from build123d import *

# Parameters (mm, degrees)
SKETCH1_R           = 1.65
BOSS_EXTRUDE1_DEPTH = 3
BOSS_EXTRUDE2_DEPTH = 16
SKETCH3_R           = 1.65
CUT_EXTRUDE1_DEPTH  = 16
SKETCH5_W           = 10
SKETCH5_H           = 3
BOSS_EXTRUDE3_DEPTH = 14
SKETCH6_R           = 1.65
CUT_EXTRUDE2_DEPTH  = 14


with BuildPart() as part:
    # Sketch1 → Boss-Extrude1 (new body)
    with BuildSketch(Plane(origin=(0, 0, 0), x_dir=(1, 0, 0), z_dir=(0, 1, 0))):
        with BuildLine():
            Line((-10, 70.842692107), (-10, 10))
            Line((-10, 10), (-70.842692107, 10))
            ThreePointArc((-70.842692107, 10), (-71.369207057, 5.012315742), (-71.545, 0))
            ThreePointArc((-71.545, 0), (50.58995466, -50.58995466), (0, 71.545))
            ThreePointArc((0, 71.545), (-5.012315742, 71.369207057), (-10, 70.842692107))
        make_face()
        with Locations((12.13, 16)):
            Circle(SKETCH1_R, mode=Mode.SUBTRACT)
        with Locations((12.13, 54)):
            Circle(SKETCH1_R, mode=Mode.SUBTRACT)
        with Locations((23.25, -21)):
            Circle(SKETCH1_R, mode=Mode.SUBTRACT)
        with Locations((-31.75, -21)):
            Circle(SKETCH1_R, mode=Mode.SUBTRACT)
    extrude(amount=BOSS_EXTRUDE1_DEPTH)

    # Sketch2 → Boss-Extrude2 (add)
    with BuildSketch(Plane.XZ):
        Polygon((-23.600230141, -61.909816502), (53.19593923, -39.496687094), (54.036431583, -42.376543445), (-22.759737789, -64.789672853), align=None)
    extrude(amount=BOSS_EXTRUDE2_DEPTH)

    # Sketch3 → Cut-Extrude1 (cut)
    with BuildSketch(Plane(origin=(14.797854544, 0, -50.703251798), x_dir=(0.959952117, 0, 0.280164118), z_dir=(-0.280164118, 0, 0.959952117))):
        with Locations((-31, -8)):
            Circle(SKETCH3_R)
        with Locations((31, -8)):
            Circle(SKETCH3_R)
    extrude(amount=-CUT_EXTRUDE1_DEPTH, mode=Mode.SUBTRACT)

    # Sketch5 → Boss-Extrude3 (add)
    with BuildSketch(Plane(origin=(0, 0, 0), x_dir=(-1, 0, 0), z_dir=(0, -1, 0))):
        with Locations((0, -63.5)):
            Rectangle(SKETCH5_W, SKETCH5_H)
    extrude(amount=BOSS_EXTRUDE3_DEPTH)

    # Sketch6 → Cut-Extrude2 (cut)
    with BuildSketch(Plane(origin=(0, 0, 62), x_dir=(-1, 0, 0), z_dir=(0, 0, -1))):
        with Locations((0, -7.998816604)):
            Circle(SKETCH6_R)
    extrude(amount=-CUT_EXTRUDE2_DEPTH, mode=Mode.SUBTRACT)


solid = part.part
Model file for the job. Use its own axes, mm. A direction names the side the tool comes from. Give positions to 0.01 mm unless a question says otherwise; leave off trailing zeros. Write each loop counter-clockwise with the first axis right and the second up, starting at its lowest first coordinate (ties: lowest second). Pieces come first, ordered by that corner, then holes. Notation, with made-up numbers: (-9, -22.75) - (17, -22.75) arc R22 cw to (17, -3.75) - close; hole circle Ø4 at (-19.5, -12.75). An arc over 180 degrees is marked (long way). Answer as CSV lines item,"result".
1. Drill centre lines: L1, parallel to Y at x = 0, z = 63; L2, parallel to X at y = 2.45, z = 21; L3, parallel to X at y = -0.25, z = 63. Where is each one in solid material? Low to high. Write a range as [from, to].
Responses:
L1,"y = [-14, -9.65], [-6.35, 3]"
L2,"x = [-68.39, -33.4], [-30.1, 21.6], [24.9, 68.39]"
L3,"x = [-5, 5]"
2. Pin check, flat tips, straight feed: pin 1 (1.5 mm diameter, centred on x = -53, y = 2, fed in from -Z); pin 2 (5.5 mm diameter, centred on x = -13.5, z = -61.5, fed in from +Y); pin 3 (1.5 mm diameter, centred on x = 40, z = -37, fed in from -Y). Stop position of each tip, or through.
Responses:
pin 1,"stops at z = -10"
pin 2,"stops at y = 0"
pin 3,"stops at y = 0"
3. Band-saw the part on D-D (z = -16). Write the cut outline in (x, y).
Responses:
outline,"(-10, 0) - (10.48, 0) - (10.48, 3) - (-10, 3) - close; (13.78, 0) - (69.73, 0) - (69.73, 3) - (13.78, 3) - close"
4. 3-axis set-ups, long thin cutter, end or side, ignore diameter. For faces 4 (the face through (-17, 0, -61)), 5 (the face through (16.176, -7.888, -53.426)), 6 (the face through (13.654, 1.479, -53.368)), 7 (the face through (0, -5, 62)), 8 (the face through (15, 3, 15)): which of +Z, -Z, +X, -X, +Y, -Y reach the whole face in a straight line?
Responses:
face 4,"-Z, -X, +Y"
face 5,"-Z, +X, -Y"
face 6,"+Y"
face 7,"+X, -X, -Y"
face 8,"+Z, -Z, +X, -X, +Y"
5. Band-saw the part on C-C (x = 49). Write the cut outline in (y, z), and give its area (3 significant figures).
Responses:
outline,"(-16, -43.85) - (0, -43.85) - (0, -52.13) - (3, -52.13) - (3, 52.13) - (0, 52.13) - (0, -40.72) - (-16, -40.72) - close"
area,"363 mm2"
6. Two-plate mould, pull along Z, no slides. Class faces 1 (the face through (1.31, -9, 63.48)), 2 (the face through (0, -5, 65)), 3 (the face through (13, 1.5, -17.4)): +Z half, -Z half, draft (parallel to the pull), parting line (faces both ways), or undercut.
Responses:
face 1,"draft"
face 2,"+Z half"
face 3,"undercut"
7. Band-saw the part on B-B (z = 21). Write the cut outline in (x, y), and give its area (3 significant figures).
Responses:
outline,"(-68.39, 0) - (-33.4, 0) - (-33.4, 3) - (-68.39, 3) - close; (-30.1, 0) - (21.6, 0) - (21.6, 3) - (-30.1, 3) - close; (24.9, 0) - (68.39, 0) - (68.39, 3) - (24.9, 3) - close"
area,"391 mm2"
8. Band-saw the part on A-A (y = -4). Write the cut outline in (x, z).
Responses:
outline,"(-23.6, -61.91) - (-22.76, -64.79) - (54.04, -42.38) - (53.2, -39.5) - close; (-5, 62) - (5, 62) - (5, 65) - (-5, 65) - close"
